```python
from build123d import *

# Parameters (mm, degrees)
SKETCH1_W           = 140
SKETCH1_H           = 45
BOSS_EXTRUDE1_DEPTH = 6


with BuildPart() as part:
    # Sketch1 → Boss-Extrude1 (new body)
    with BuildSketch(Plane.XY):
        with Locations((70, 22.5)):
            Rectangle(SKETCH1_W, SKETCH1_H)
        with BuildLine():
            Line((26.683203231, 24), (113.316796769, 24))
            ThreePointArc((113.316796769, 24), (114.816796769, 22.5), (113.316796769, 21))
            Line((113.316796769, 21), (26.683203231, 21))
            ThreePointArc((26.683203231, 21), (25.183203231, 22.5), (26.683203231, 24))
        make_face(mode=Mode.SUBTRACT)
        with BuildLine():
            Line((26.683203231, 35.803698148), (113.316796769, 35.803698148))
            ThreePointArc((113.316796769, 35.803698148), (114.816796769, 34.303698148), (113.316796769, 32.803698148))
            Line((113.316796769, 32.803698148), (26.683203231, 32.803698148))
            ThreePointArc((26.683203231, 32.803698148), (25.183203231, 34.303698148), (26.683203231, 35.803698148))
        make_face(mode=Mode.SUBTRACT)
        with BuildLine():
            Line((26.683203231, 12.405318703), (113.316796769, 12.405318703))
            ThreePointArc((113.316796769, 12.405318703), (114.816796769, 10.905318703), (113.316796769, 9.405318703))
            Line((113.316796769, 9.405318703), (26.683203231, 9.405318703))
            ThreePointArc((26.683203231, 9.405318703), (25.183203231, 10.905318703), (26.683203231, 12.405318703))
        make_face(mode=Mode.SUBTRACT)
    extrude(amount=BOSS_EXTRUDE1_DEPTH)


solid = part.part
```
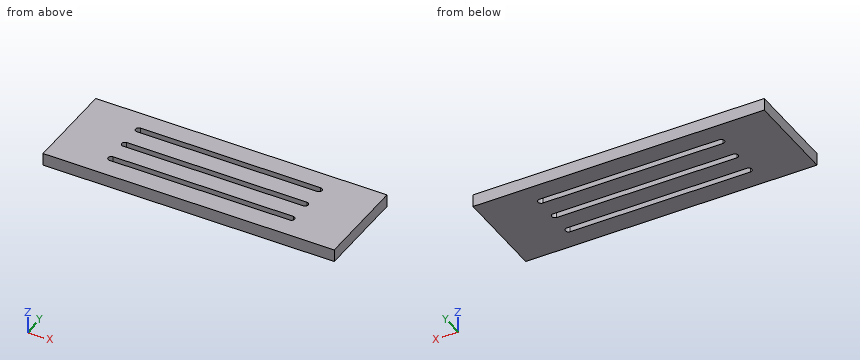
Work out the finished part from the listing and answer in its coordinate system (mm). Give positions to 0.01 mm unless a question says otherwise; leave off trailing zeros. Order: outer loops, then holes, each group sorted by start corner. A loop starts at its lowest first (then second) coordinate and runs counter-clockwise, first axis right, second up. Notation, with made-up numbers: (35, 7.5) -> (58, 7.5) arc R28 ccw to (58, 37.5) -> close; hole circle Ø2 at (45, 23.5). An arc over 180 degrees is marked (long way). Answer as CSV lines item,"result". Start each with the question number.
(1) Section A-A, the plane y = 22.5 is taken. Write down the section's boundary in (x, z).
(2) Section C-C, the plane x = 38.5 is taken. Write down the section's boundary in (y, z), plus the area to 3 significant figures.
(3) Consider line 1 along Y through (x, z) = (104, 2.2); line 2 along X through (y, z) = (22.5, 5.3); line 3 along X through (y, z) = (35.5, 1.6). Determine where each line is inside the solid, lowest interval first.
(4) Section B-B, the plane z = 3.1 is taken. Write down the section's boundary in (x, y), plus the area to 3 significant figures.
Entries:
1,outline,"(0, 0) -> (25.18, 0) -> (25.18, 6) -> (0, 6) -> close; (114.82, 0) -> (140, 0) -> (140, 6) -> (114.82, 6) -> close"
2,outline,"(0, 0) -> (9.41, 0) -> (9.41, 6) -> (0, 6) -> close; (12.41, 0) -> (21, 0) -> (21, 6) -> (12.41, 6) -> close; (24, 0) -> (32.8, 0) -> (32.8, 6) -> (24, 6) -> close; (35.8, 0) -> (45, 0) -> (45, 6) -> (35.8, 6) -> close"
2,area,"216 mm²"
3,line 1,"0 to 9.41, 12.41 to 21, 24 to 32.8, 35.8 to 45"
3,line 2,"0 to 25.18, 114.82 to 140"
3,line 3,"0 to 25.78, 114.22 to 140"
4,outline,"(0, 0) -> (140, 0) -> (140, 45) -> (0, 45) -> close; hole (26.68, 9.41) -> (113.32, 9.41) arc R1.5 ccw to (113.32, 12.41) -> (26.68, 12.41) arc R1.5 ccw to start; hole (26.68, 21) -> (113.32, 21) arc R1.5 ccw to (113.32, 24) -> (26.68, 24) arc R1.5 ccw to start; hole (26.68, 32.8) -> (113.32, 32.8) arc R1.5 ccw to (113.32, 35.8) -> (26.68, 35.8) arc R1.5 ccw to start"
4,area,"5,500 mm²"
